```python
from build123d import *

# Parameters (mm, degrees)
F1_DEPTH = 63.5
F0_W     = 50.8
F0_H     = 19.05
F2_DEPTH = 25.4
F3_DEPTH = 7.9375


with BuildPart() as f1:
    # F0 (on Front) → F1 (new body, symmetric)
    with BuildSketch(Plane.XZ):
        Polygon((41.275, -9.525), (41.275, 9.525), (22.225, 9.525), (-41.275, 9.525), (-41.275, -9.525), align=None)
    extrude(amount=F1_DEPTH, both=True)

    # F0 (on Front) → F2 (join, symmetric)
    with BuildSketch(Plane.XZ):
        with BuildLine():
            Line((22.225, 9.525), (41.275, 9.525))
            Line((41.275, 9.525), (41.275, 27.0002))
            ThreePointArc((41.275, 27.0002), (45.9246798487, 38.2255201513), (57.15, 42.8752))
            Line((57.15, 42.8752), (60.325, 42.8752))
            Line((60.325, 42.8752), (60.325, 61.9252))
            Line((60.325, 61.9252), (57.15, 61.9252))
            ThreePointArc((57.15, 61.9252), (32.4542956671, 51.6959043329), (22.225, 27.0002))
            Line((22.225, 27.0002), (22.225, 9.525))
        make_face()
        with Locations((85.725, 52.4002)):
            Rectangle(F0_W, F0_H)
    extrude(amount=F2_DEPTH, both=True)

    # F0 (on Front) → F3 (join, symmetric)
    with BuildSketch(Plane.XZ):
        with BuildLine():
            Line((-41.275, 9.525), (22.225, 9.525))
            Line((22.225, 9.525), (22.225, 27.0002))
            ThreePointArc((22.225, 27.0002), (32.4542956671, 51.6959043329), (57.15, 61.9252))
            add(Edge.make_bspline(
                [(-41.275, 9.525), (-39.5729020238, 63.4139552712), (19.462088123, 63.0895867944), (57.15, 61.9252)],
                knots=[0, 0, 0, 0, 111.5045361635, 111.5045361635, 111.5045361635, 111.5045361635], degree=3))
        make_face()
    extrude(amount=F3_DEPTH, both=True)


solid = f1.part
```
Read the model definition and answer for the solid it produces. Units are mm, in the model's axes. A direction names the side the tool comes from. Round coordinates to 2 decimals unless told otherwise and drop trailing zeros. Write each loop counter-clockwise with the first axis right and the second up, starting at its lowest first coordinate (ties: lowest second). Pieces come first, ordered by that corner, then holes. Notation, with made-up numbers: (83, -8.5) - (128, -8.5) arc R30 ccw to (128, 20.5) - close; hole circle Ø2 at (0, 5.25). An arc over 180 degrees is marked (long way). Use CSV: the item, a comma, the result in double quotes.
Q1. Determine the mould class of faces 6 (the flat face through (-4, 7.938, 37)), 7 (the flat face through (-1, -63.5, 0)), 8 (the flat face through (41.275, -1, 4)) for opening direction Y: +Y half, -Y half, draft (parallel to the pull), parting line (faces both ways), or undercut.
Values:
face 6,"+Y half"
face 7,"-Y half"
face 8,"draft"
Q2. Find section A-A, the plane y = -23. Write down the section's boundary in (x, z) (3 decimals), then the cut area to 3 significant figures.
Values:
outline,"(-41.275, -9.525) - (41.275, -9.525) - (41.275, 27) arc R15.875 cw to (57.15, 42.875) - (111.125, 42.875) - (111.125, 61.925) - (57.15, 61.925) arc R34.925 ccw to (22.225, 27) - (22.225, 9.525) - (-41.275, 9.525) - close"
area,"3,690 mm²"
Q3. Straight lines are drawn through the part: line 1 along Y through (x, z) = (12, 56); line 2 along Z through (x, y) = (57.5, 9); line 3 along X through (y, z) = (56, -5) (3 decimals). For each, find the intervals that lie inside material, in ascending order.
Values:
line 1,"y = -7.94 to 7.94"
line 2,"z = 42.88 to 61.93"
line 3,"x = -41.275 to 41.275"
Q4. Each of these flat-tipped pins is pushed along its axis until it touches: pin 1 Ø1 at (x, z) = (24.5, 16) entering from +Y; pin 2 Ø19 at (y, z) = (-18.5, 21) entering from -X (3 decimals); pin 3 Ø4 at (x, z) = (-18.5, 16) entering from +Y. Where does it stop, or does it pass through?
Values:
pin 1,"stops at y = 25.4"
pin 2,"stops at x = 22.225"
pin 3,"stops at y = 7.94"
Q5. A tool of negligible diameter and unlimited length cuts with its end or side. For faces 1 (the flat face through (-4, -7.938, 37)), 2 (the flat face through (85, 0, 61.925)), 3 (the flat face through (84, 0, 42.875)), 4 (the cylindrical face through (32.73, 16.55, 51.97)), 5 (the flat face through (56, -25.4, 48)), from which of +Z, -Z, +X, -X, +Y, -Y can it reach the whole face along a straight path? Write none if from no direction.
Values:
face 1,"+Z, -X, -Y"
face 2,"+Z, +X, +Y, -Y"
face 3,"-Z, +X, +Y, -Y"
face 4,"+Z, -X, +Y"
face 5,"+Z, +X, -X, -Y"
Q6. Find section B-B, the plane z = -2.5. Write down the section's boundary in (x, y) (3 decimals).
Values:
outline,"(-41.275, -63.5) - (41.275, -63.5) - (41.275, 63.5) - (-41.275, 63.5) - close"
Q7. Find section C-C, the plane x = 102. Write down the section's boundary in (y, z).
Values:
outline,"(-25.4, 42.88) - (25.4, 42.88) - (25.4, 61.93) - (-25.4, 61.93) - close"
